```python
from build123d import *

# Parameters (mm, degrees)
SKETCH1_W           = 39.999999999
SKETCH1_H           = 30
BOSS_EXTRUDE1_DEPTH = 30
SKETCH2_W           = 17.2
SKETCH2_H           = 33.728920846
CUT_EXTRUDE1_DEPTH  = 25
SKETCH3_R           = 3
CUT_EXTRUDE2_DEPTH  = 77.38910698
SKETCH4_W           = 8.5
SKETCH4_H           = 4.5
SKETCH4_W_2         = 4.5
SKETCH4_H_2         = 8.5
CUT_EXTRUDE3_DEPTH  = 9
CUT_EXTRUDE4_START  = -40
SKETCH4_2_W         = 8.5
SKETCH4_2_H         = 4.5
SKETCH4_2_W_2       = 4.5
SKETCH4_2_H_2       = 8.5
CUT_EXTRUDE4_DEPTH  = 9
SKETCH5_R           = 2.5
CUT_EXTRUDE5_DEPTH  = 12
CHAMFER1_SIZE       = 4
SKETCH6_R           = 5
CUT_EXTRUDE6_DEPTH  = 8
CUT_EXTRUDE7_DEPTH  = 8


with BuildPart() as part:
    # Sketch1 → Boss-Extrude1 (new body)
    with BuildSketch(Plane.XY):
        with Locations((-51.592932584, 42.752018711)):
            Rectangle(SKETCH1_W, SKETCH1_H)
    extrude(amount=BOSS_EXTRUDE1_DEPTH)

    # Sketch2 → Cut-Extrude1 (cut)
    with BuildSketch(Plane(origin=(0, 57.752018711, 0), x_dir=(1, 0, 0), z_dir=(0, 1, 0))):
        with Locations((-51.872932582, -8.135539577)):
            Rectangle(SKETCH2_W, SKETCH2_H)
    extrude(amount=-CUT_EXTRUDE1_DEPTH, mode=Mode.SUBTRACT)

    # Sketch3 → Cut-Extrude2 (cut, through all)
    with BuildSketch(Plane(origin=(-31.592932584, 0, 0), x_dir=(0, 0, -1), z_dir=(1, 0, 0))):
        with Locations((-12.822072937, 44.929945774)):
            Circle(SKETCH3_R)
    extrude(amount=-CUT_EXTRUDE2_DEPTH, mode=Mode.SUBTRACT)

    # Sketch4 → Cut-Extrude3 (cut)
    with BuildSketch(Plane(origin=(-31.592932584, 0, 0), x_dir=(0, 0, -1), z_dir=(1, 0, 0))):
        with Locations((-9.25, 35.002018711)):
            Rectangle(SKETCH4_W, SKETCH4_H)
        with Locations((-22.75, 48.502018711)):
            Rectangle(SKETCH4_W_2, SKETCH4_H_2)
    extrude(amount=-CUT_EXTRUDE3_DEPTH, mode=Mode.SUBTRACT)

    # Sketch4<2> → Cut-Extrude4 (cut)
    with BuildSketch(Plane(origin=(-31.592932584, 0, 0), x_dir=(0, 0, -1), z_dir=(1, 0, 0)).offset(CUT_EXTRUDE4_START)):
        with Locations((-9.25, 35.002018711)):
            Rectangle(SKETCH4_2_W, SKETCH4_2_H)
        with Locations((-22.75, 48.502018711)):
            Rectangle(SKETCH4_2_W_2, SKETCH4_2_H_2)
    extrude(amount=CUT_EXTRUDE4_DEPTH, mode=Mode.SUBTRACT)

    # Sketch5 → Cut-Extrude5 (cut)
    with BuildSketch(Plane.XY.offset(30)):
        with Locations((-66.592932583, 48.502018711)):
            Circle(SKETCH5_R)
        with Locations((-36.592932584, 48.502018711)):
            Circle(SKETCH5_R)
    cut_extrude5 = extrude(amount=-CUT_EXTRUDE5_DEPTH, mode=Mode.SUBTRACT)

    # Mirror1: Cut-Extrude5 across plane
    add(cut_extrude5.mirror(Plane(origin=(0, 28.876009355, 28.876009355), x_dir=(0, -0.7071067811865478, 0.7071067811865472), z_dir=(0, -0.7071067811865475, -0.7071067811865477))), mode=Mode.SUBTRACT)

    # Chamfer1
    chamfer1_edges = [part.edges().sort_by_distance(p)[0] for p in [
        (-51.592932584, 27.752018711, 30),
        (-66.032932583, 57.752018711, 0),
        (-51.592932584, 27.752018711, 0),
        (-37.432932583, 57.752018711, 0),
        (-51.592932584, 57.752018711, 30),
    ]]
    chamfer(chamfer1_edges, length=CHAMFER1_SIZE)

    # Sketch6 → Cut-Extrude6 (cut)
    with BuildSketch(Plane(origin=(-31.592932584, 0, 0), x_dir=(0, 0, -1), z_dir=(1, 0, 0))):
        with Locations((-12.822072937, 44.929945774)):
            Circle(SKETCH6_R)
    extrude(amount=-CUT_EXTRUDE6_DEPTH, mode=Mode.SUBTRACT)

    # Sketch7 → Cut-Extrude7 (cut)
    with BuildSketch(Plane.ZY.offset(71.592932583)):
        Polygon((15.304679094, 40.629945774), (17.787285252, 44.929945774), (15.304679094, 49.229945774), (10.339466779, 49.229945774), (7.856860622, 44.929945774), (10.339466779, 40.629945774), align=None)
    extrude(amount=-CUT_EXTRUDE7_DEPTH, mode=Mode.SUBTRACT)


solid = part.part
```
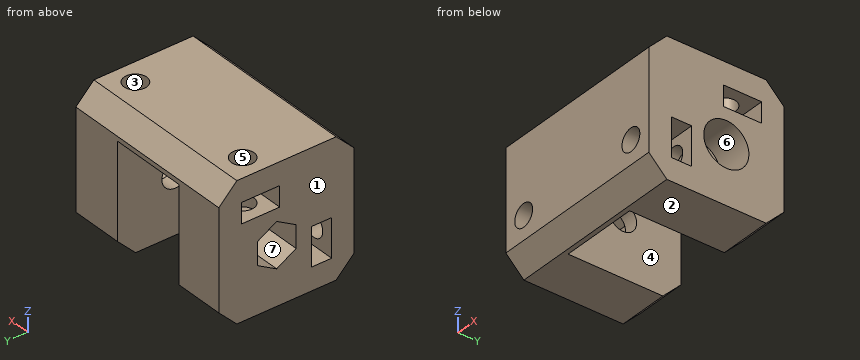
Could you check a few things on this model? Use its own coordinates, in mm. Face numbers are marked on the shaded views. A direction names the side the tool comes from. Give positions to 0.01 mm unless a question says otherwise; leave off trailing zeros. Write each loop counter-clockwise with the first axis right and the second up, starting at its lowest first coordinate (ties: lowest second). Pieces come first, ordered by that corner, then holes. Notation, with made-up numbers: (78, 3.5) - (107, 3.5) arc R9 cw to (107, 16.5) - close; hole circle Ø4 at (2, -34.75). An arc over 180 degrees is marked (long way). One line per item, written item: value. Start each with the question number.
Item 1: Please list where these lines run through material, in increasing order: line 1 (X direction, y = 39.15, z = 9.25); line 2 (X direction, y = 35, z = 18); line 3 (X direction, y = 33, z = 9). Write a range as from..to.
Item 2: I'm going to push flat-ended pins straight in: pin 1 (1 mm diameter, centred on x = -54, z = 17.5, fed in from +Y); pin 2 (5 mm diameter, centred on y = 44.93, z = 12.82, fed in from +X); pin 3 (2 mm diameter, centred on x = -67, z = 10, fed in from -Y); pin 4 (3 mm diameter, centred on y = 45.5, z = 10, fed in from +X). Where does each tip first touch, or does it pass through?
Item 3: If we mould it in two halves opening along X, with no side actions, what happens to the marked faces 1, 2 and 3? For each: +X half, -X half, draft (parallel to the pull), parting line (faces both ways), or undercut.
Item 4: Imagine slicing it at A-A, the plane x = -33.5. List the corners of the cut face in (y, z) for me.
Item 5: Imagine slicing it at C-C, the plane x = -42.5. List the corners of the cut face in (y, z) for me.
Item 6: Imagine slicing it at B-B, the plane y = 35.5. List the corners of the cut face in (x, z) for me.
Item 7: Imagine slicing it at D-D, the plane x = -57. List the corners of the cut face in (y, z) for me, and give its area (3 significant figures).
Item 8: Which directions (+Z, -Z, +X, -X, +Y, -Y) give clear straight access to the entire face, cutting with the end or side of a thin tool? Please do the marked faces 4, 5, 6 and 7.
Geometry says:
1. line 1: -71.59..-69.09, -64.09..-60.47, -43.27..-39.09, -34.09..-31.59
1. line 2: -71.59..-60.47, -43.27..-31.59
1. line 3: -62.59..-60.47, -43.27..-40.59
2. pin 1: y = 32.75
2. pin 2: through
2. pin 3: y = 39.75
2. pin 4: x = -39.59
3. face 1: -X half
3. face 2: draft
3. face 3: undercut
4. outline: (27.75, 4) - (31.75, 0) - (53.75, 0) - (57.75, 4) - (57.75, 26) - (53.75, 30) - (31.75, 30) - (27.75, 26) - close; hole (32.75, 5) - (37.25, 5) - (37.25, 13.5) - (32.75, 13.5) - close; hole circle Ø10 at (44.93, 12.82); hole (44.25, 20.5) - (52.75, 20.5) - (52.75, 25) - (44.25, 25) - close
5. outline: (27.75, 4) - (31.75, 0) - (53.75, 0) - (57.75, 4) - (57.75, 26) - (53.75, 30) - (31.75, 30) - (27.75, 26) - close; hole circle Ø6 at (44.93, 12.82)
6. outline: (-71.59, 0) - (-60.47, 0) - (-60.47, 25) - (-43.27, 25) - (-43.27, 0) - (-31.59, 0) - (-31.59, 5) - (-40.59, 5) - (-40.59, 13.5) - (-31.59, 13.5) - (-31.59, 30) - (-71.59, 30) - (-71.59, 13.5) - (-62.59, 13.5) - (-62.59, 5) - (-71.59, 5) - close
7. outline: (27.75, 4) - (31.75, 0) - (32.75, 0) - (32.75, 25) - (57.75, 25) - (57.75, 26) - (53.75, 30) - (31.75, 30) - (27.75, 26) - close
7. area: 251 mm^2
8. face 4: -Z, +Y
8. face 5: +Z
8. face 6: +X
8. face 7: -X
